Verification items for the finished model (mm, model axes). Round coordinates to 2 decimals unless told otherwise and drop trailing zeros. Loops run counter-clockwise (first coordinate to the right, second up) from the corner with the lowest first, then second, coordinate; pieces in that order, holes last. Notation, with made-up numbers: (-17, 17) -> (-1, 17) arc R18 cw to (-1, 39) -> close; hole circle Ø7 at (-24, -31.75). An arc over 180 degrees is marked (long way). Use CSV: the item, a comma, the result in double quotes. Start each with the question number.
```python
from build123d import *

# Parameters (mm, degrees)
SKETCH1_W           = 101.6
SKETCH1_H           = 101.6
BOSS_EXTRUDE1_DEPTH = 2.54
SKETCH3_R           = 4.191
CUT_EXTRUDE2_DEPTH  = 2.54
SKETCH2_R           = 4.826
CUT_EXTRUDE3_DEPTH  = 2.54


with BuildPart() as part:
    # Sketch1 → Boss-Extrude1 (new body)
    with BuildSketch(Plane.XY):
        Rectangle(SKETCH1_W, SKETCH1_H)
    extrude(amount=BOSS_EXTRUDE1_DEPTH)

    # Sketch3 → Cut-Extrude2 (cut)
    with BuildSketch(Plane.XY.offset(2.54)):
        Circle(SKETCH3_R)
    extrude(amount=-CUT_EXTRUDE2_DEPTH, mode=Mode.SUBTRACT)

    # Sketch2 → Cut-Extrude3 (cut)
    with BuildSketch(Plane.XY.offset(2.54)):
        with Locations((-44.45, 44.45)):
            Circle(SKETCH2_R)
        with Locations((44.45, 44.45)):
            Circle(SKETCH2_R)
        with Locations((44.45, -44.45)):
            Circle(SKETCH2_R)
        with Locations((-44.190779842, -44.45)):
            Circle(SKETCH2_R)
    extrude(amount=-CUT_EXTRUDE3_DEPTH, mode=Mode.SUBTRACT)


solid = part.part
```
Q1. Cross-section at B-B (x = 42.5). Record the boundary of the cut face in (y, z), and give its area (3 significant figures).
Q2. Cross-section at A-A (y = 0). Record the boundary of the cut face in (x, z), and give its area (3 significant figures).
Q3. Cross-section at D-D (z = 1.9). Record the boundary of the cut face in (x, y), and give its area (3 significant figures).
Q4. Release check for a two-part mould opening along X. For faces 1 (the face through (50.8, -1, 1)), 2 (the face through (11, 1, 0)), 3 (the face through (-49.012, -44.238, 1.288)) record: +X half, -X half, draft (parallel to the pull), parting line (faces both ways), or undercut.
Q5. Depth check by flat-ended pin: pin 1 Ø5 at (x, y) = (24, 40) entering from -Z; pin 2 Ø6 at (x, y) = (-44.45, 44.45) entering from +Z. Enter the tip coordinate at first touch or a pass-through.
Q6. Thickness scan on L1, parallel to Y at x = 44.45, z = 0.9; L2, parallel to Y at x = 0, z = 2.05; L3, parallel to Y at x = -40, z = 0.2. Record the ranges inside material, lowest first. Write a range as from..to.
Answer list:
1,outline,"(-50.8, 0) -> (-48.86, 0) -> (-48.86, 2.54) -> (-50.8, 2.54) -> close; (-40.04, 0) -> (40.04, 0) -> (40.04, 2.54) -> (-40.04, 2.54) -> close; (48.86, 0) -> (50.8, 0) -> (50.8, 2.54) -> (48.86, 2.54) -> close"
1,area,"213 mm2"
2,outline,"(-50.8, 0) -> (-4.19, 0) -> (-4.19, 2.54) -> (-50.8, 2.54) -> close; (4.19, 0) -> (50.8, 0) -> (50.8, 2.54) -> (4.19, 2.54) -> close"
2,area,"237 mm2"
3,outline,"(-50.8, -50.8) -> (50.8, -50.8) -> (50.8, 50.8) -> (-50.8, 50.8) -> close; hole circle Ø9.65 at (-44.45, 44.45); hole circle Ø9.65 at (-44.19, -44.45); hole circle Ø8.38 at (0, 0); hole circle Ø9.65 at (44.45, -44.45); hole circle Ø9.65 at (44.45, 44.45)"
3,area,"9,970 mm2"
4,face 1,"+X half"
4,face 2,"draft"
4,face 3,"undercut"
5,pin 1,"stops at z = 0"
5,pin 2,"passes through"
6,L1,"y = -50.8..-49.28, -39.62..39.62, 49.28..50.8"
6,L2,"y = -50.8..-4.19, 4.19..50.8"
6,L3,"y = -50.8..-46.84, -42.06..42.58, 46.32..50.8"
